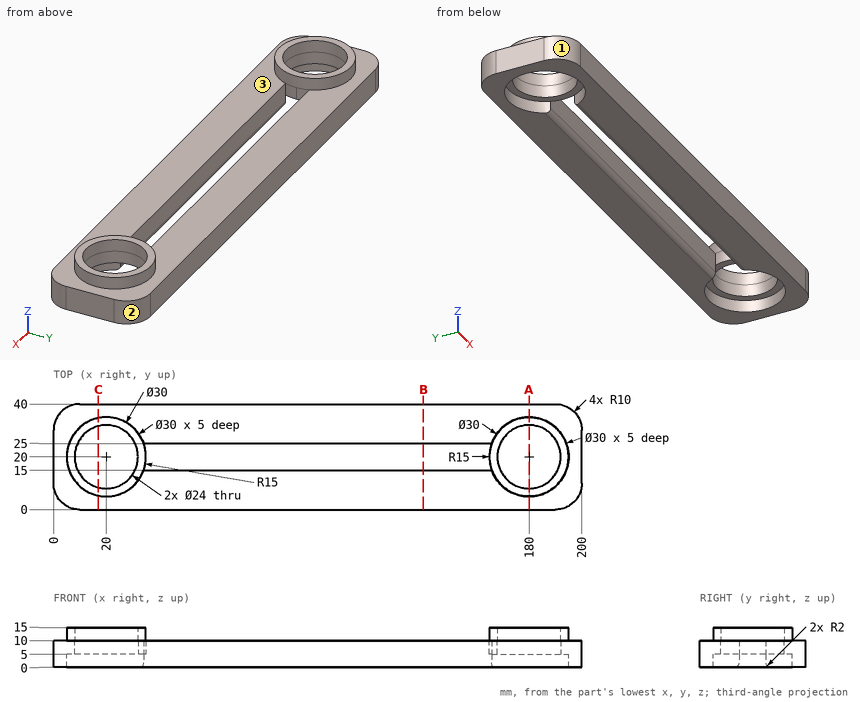
Check sheet for the drawn part. Datum: minimum x, y, z corner. Units: mm. Round coordinates to 2 decimals unless told otherwise and drop trailing zeros. Loops run counter-clockwise (first coordinate to the right, second up) from the corner with the lowest first, then second, coordinate; pieces in that order, holes last. Notation, with made-up numbers: (86, -3.75) - (95, -3.75) arc R3 cw to (95, 0.25) - close; hole circle Ø6 at (53, 40.25). An arc over 180 degrees is marked (long way). Answer as a JSON object with one key per item and string values. Group by question number.
Q1. Scan lines: line 1 along Y through (x, z) = (78, 2.25); line 2 along X through (y, z) = (12, 2.5); line 3 along Y through (x, z) = (180, 8.05). Record each from-to range of solid material in increasing order. Write a range as [from, to].
Q2. Mould release check, pull along X, two halves, no side actions. Record for the marked faces 1, 2 and 3: released by +X, released by -X, zero draft, split by the parting line, or undercut.
Q3. Sectioned sample at A-A, the plane x = 180. Enter the section's corners in (y, z), plus the area to 3 significant figures.
Q4. Sectioned sample at B-B, the plane x = 140. Enter the section's corners in (y, z).
Q5. Sectioned sample at C-C, the plane x = 17. Enter the section's corners in (y, z).
Q6. Gauge pin test, flat ends, axial feed: P1, Ø19, axis at x = 180, y = 20, coming from the -Z side; P2, Ø1.5, axis at x = 101, y = 11, coming from the +Z side; P3, Ø5, axis at y = 33.5, z = 5, coming from the +X side; P4, Ø1, axis at y = 35, z = 4.5, coming from the +X side. Record the tip position at first contact, or that the pin passes through.
Solution:
{
 "1": {"line 1": "y = [0, 15], [25, 40]", "line 2": "x = [0, 7.31], [32.69, 167.31], [192.69, 200]", "line 3": "y = [0, 8], [32, 40]"},
 "2": {"face 1": "released by -X", "face 2": "released by +X", "face 3": "undercut"},
 "3": {"outline": "(0, 0) - (5, 0) - (5, 5) - (8, 5) - (8, 15) - (5, 15) - (5, 10) - (0, 10) - close; (32, 5) - (35, 5) - (35, 0) - (40, 0) - (40, 10) - (35, 10) - (35, 15) - (32, 15) - close", "area": "160 mm²"},
 "4": {"outline": "(0, 0) - (13, 0) arc R2 ccw to (15, 2) - (15, 10) - (0, 10) - close; (25, 2) arc R2 ccw to (27, 0) - (40, 0) - (40, 10) - (25, 10) - close"},
 "5": {"outline": "(0, 0) - (5.3, 0) - (5.3, 5) - (8.38, 5) - (8.38, 15) - (5.3, 15) - (5.3, 10) - (0, 10) - close; (31.62, 5) - (34.7, 5) - (34.7, 0) - (40, 0) - (40, 10) - (34.7, 10) - (34.7, 15) - (31.62, 15) - close"},
 "6": {"P1": "passes through", "P2": "stops at z = 10", "P3": "stops at x = 199.95", "P4": "stops at x = 198.93"}
}
